Design review of the part built by this model. Coordinates are the model's own, in mm. A direction names the side the tool comes from. Give positions to 0.01 mm unless a question says otherwise; leave off trailing zeros. Write each loop counter-clockwise with the first axis right and the second up, starting at its lowest first coordinate (ties: lowest second). Pieces come first, ordered by that corner, then holes. Notation, with made-up numbers: (88.25, 37.25) - (137.25, 37.25) arc R13 cw to (137.25, 60.25) - close; hole circle Ø2 at (-8, -32.75). An arc over 180 degrees is marked (long way). Use a Markdown table: item, result. Add a question column.
```python
from build123d import *

# Parameters (mm, degrees)
SKETCH2_W           = 6
SKETCH2_H           = 5
BOSS_EXTRUDE1_DEPTH = 9
SKETCH3_R           = 1.9
SKETCH3_R_2         = 0.6
CUT_EXTRUDE1_DEPTH  = 7
FILLET1_R           = 0.6
SKETCH4_W           = 0.5
SKETCH4_H           = 1.2
BOSS_EXTRUDE2_DEPTH = 3
FILLET2_R           = 0.6
SKETCH5_R           = 0.65
BOSS_EXTRUDE3_DEPTH = 1
FILLET3_R           = 0.1
SKETCH6_R           = 1
CUT_EXTRUDE2_DEPTH  = 0.2


with BuildPart() as part:
    # Sketch2 → Boss-Extrude1 (new body)
    with BuildSketch(Plane(origin=(0, 0, 0), x_dir=(1, 0, 0), z_dir=(0, 1, 0))):
        Rectangle(SKETCH2_W, SKETCH2_H)
    extrude(amount=BOSS_EXTRUDE1_DEPTH)

    # Sketch3 → Cut-Extrude1 (cut)
    with BuildSketch(Plane(origin=(0, 9, 0), x_dir=(1, 0, 0), z_dir=(0, 1, 0))):
        with Locations(Location((0.5, 0, 0), (0, 0, 270))):
            Circle(SKETCH3_R)
        with Locations(Location((0.5, 0, 0), (0, 0, 270))):
            Circle(SKETCH3_R_2, mode=Mode.SUBTRACT)
    extrude(amount=-CUT_EXTRUDE1_DEPTH, mode=Mode.SUBTRACT)

    # Fillet1
    fillet1_edges = [part.edges().sort_by_distance(p)[0] for p in [
        (0.5, 9, -0.6),
    ]]
    fillet(fillet1_edges, radius=FILLET1_R)

    # Sketch4 → Boss-Extrude2 (add)
    with BuildSketch(Plane.XY.offset(2.5)):
        with Locations((2, 1)):
            Rectangle(SKETCH4_W, SKETCH4_H)
        with Locations((0, 1)):
            Rectangle(SKETCH4_W, SKETCH4_H)
        with Locations((-2, 1)):
            Rectangle(SKETCH4_W, SKETCH4_H)
    extrude(amount=BOSS_EXTRUDE2_DEPTH)

    # Fillet2
    fillet2_edges = [part.edges().sort_by_distance(p)[0] for p in [
        (-2, 0.4, 5.5),
        (-2, 1.6, 5.5),
        (0, 1.6, 5.5),
        (0, 0.4, 5.5),
        (2, 0.4, 5.5),
        (2, 1.6, 5.5),
    ]]
    fillet(fillet2_edges, radius=FILLET2_R - 0.0001)  # a hair under: the kernel refuses the full size

    # Sketch5 → Boss-Extrude3 (add)
    with BuildSketch(Plane.XY.offset(2.5)):
        with Locations(Location((2, 7, 0), (0, 0, 180))):
            Circle(SKETCH5_R)
        with Locations(Location((-2, 7, 0), (0, 0, 180))):
            Circle(SKETCH5_R)
    extrude(amount=BOSS_EXTRUDE3_DEPTH)

    # Fillet3
    fillet3_edges = [part.edges().sort_by_distance(p)[0] for p in [
        (2.65, 7, 3.5),
        (-1.35, 7, 3.5),
    ]]
    fillet(fillet3_edges, radius=FILLET3_R)

    # Sketch6 → Cut-Extrude2 (cut)
    with BuildSketch(Plane.XY.offset(2.5)):
        with Locations((0, 4.5)):
            Circle(SKETCH6_R)
    extrude(amount=-CUT_EXTRUDE2_DEPTH, mode=Mode.SUBTRACT)


solid = part.part
```
(1) Tool access review of faces 5 (the face through (-0.25, 1, 4)), 6 (the face through (1.75, 1, 4)), 7 (the face through (2.085, 6.356, 2.944)), 8 (the face through (2, 7, 3.5)), 9 (the face through (2.25, 1, 4)): name each direction out of +Z, -Z, +X, -X, +Y, -Y from which nothing blocks a thin tool from reaching the whole face with its end or side.
(2) Insertion check: pin 1 (1 mm diameter, centred on y = 1, z = 4, fed in from +X); pin 2 (3 mm diameter, centred on x = 0.5, y = 6, fed in from +Z); pin 3 (0.6 mm diameter, centred on y = 1, z = 4, fed in from -X). Each pin has a flat end and moves straight along its axis. Give the tip position at first contact, or say it passes through.
(3) For line 1 along X through (y, z) = (5.25, 0); line 2 along X through (y, z) = (1.5, 3.5); line 3 along Y through (x, z) = (0, 2.4), list the stretches that pass through material, from the lowest coordinate up.
(4) Add section B-B (z = 2.75). State the section outline as (x, y) points.
(5) Add section A-A (y = 4.5). State the section outline as (x, z) points, and give its area (3 significant figures).
(6) Mouldability with a two-part tool opening along X and no side actions: class faces 1 (the face through (-0.71, 5.44, 2.5)), 2 (the face through (3, 4, 0)), 3 (the face through (-2.25, 1, 4)), 4 (the face through (0, 4, -2.5)) as +X half, -X half, draft (parallel to the pull), parting line (faces both ways), or undercut.
(7) Add section C-C (y = 7). State the section outline as (x, z) points, and give its area (3 significant figures).
Answers follow:
| question | item | result |
|---|---|---|
| 1 | face 5 | +Z, +Y, -Y |
| 1 | face 6 | +Z, -Y |
| 1 | face 7 | +Z |
| 1 | face 8 | +Z, +X, -X, +Y |
| 1 | face 9 | +Z, +X, -Y |
| 2 | pin 1 | x = 2.25 |
| 2 | pin 2 | z = 3.5 |
| 2 | pin 3 | x = -2.25 |
| 3 | line 1 | -3 to -1.4, -0.1 to 1.1, 2.4 to 3 |
| 3 | line 2 | -2.25 to -1.75, -0.25 to 0.25, 1.75 to 2.25 |
| 3 | line 3 | 0 to 3.5, 5.5 to 9 |
| 4 | outline | circle Ø1.3 at (-2, 7); (-2.25, 0.4) - (-1.75, 0.4) - (-1.75, 1.6) - (-2.25, 1.6) - close; (-0.25, 0.4) - (0.25, 0.4) - (0.25, 1.6) - (-0.25, 1.6) - close; circle Ø1.3 at (2, 7); (1.75, 0.4) - (2.25, 0.4) - (2.25, 1.6) - (1.75, 1.6) - close |
| 5 | outline | (-3, -2.5) - (3, -2.5) - (3, 2.5) - (1, 2.5) - (1, 2.3) - (-1, 2.3) - (-1, 2.5) - (-3, 2.5) - close; circle Ø1.2 at (0.5, 0); hole circle Ø3.8 at (0.5, 0) |
| 5 | area | 19.4 mm^2 |
| 6 | face 1 | undercut |
| 6 | face 2 | +X half |
| 6 | face 3 | -X half |
| 6 | face 4 | draft |
| 7 | outline | (-3, -2.5) - (3, -2.5) - (3, 2.5) - (2.65, 2.5) - (2.65, 3.4) arc R0.1 ccw to (2.55, 3.5) - (1.45, 3.5) arc R0.1 ccw to (1.35, 3.4) - (1.35, 2.5) - (-1.35, 2.5) - (-1.35, 3.4) arc R0.1 ccw to (-1.45, 3.5) - (-2.55, 3.5) arc R0.1 ccw to (-2.65, 3.4) - (-2.65, 2.5) - (-3, 2.5) - close; circle Ø1.2 at (0.5, 0); hole circle Ø3.8 at (0.5, 0) |
| 7 | area | 22.4 mm^2 |
